```python
from build123d import *

# Parameters (mm, degrees)
F0_W     = 105
F0_H     = 85
F0_R     = 4
F1_DEPTH = 8
F2_D     = 9
F2_DEPTH = 14
F2_TIP   = 2.7038727856


with BuildPart() as f1:
    # F0 (on Top) → F1 (new body)
    with BuildSketch(Plane.XY):
        Rectangle(F0_W, F0_H)
        with Locations((-42.5, -30)):
            Circle(F0_R, mode=Mode.SUBTRACT)
        with Locations((42.5, -30)):
            Circle(F0_R, mode=Mode.SUBTRACT)
        with Locations((-42.5, 30)):
            Circle(F0_R, mode=Mode.SUBTRACT)
        with Locations((42.5, 30)):
            Circle(F0_R, mode=Mode.SUBTRACT)
        with Locations((-42.5, 30)):
            Circle(F0_R)
        with Locations((42.5, 30)):
            Circle(F0_R)
        with Locations((42.5, -30)):
            Circle(F0_R)
        with Locations((-42.5, -30)):
            Circle(F0_R)
    extrude(amount=F1_DEPTH)

    # F2
    with Locations(Plane(origin=(0, 0, 0), x_dir=(1, 0, 0), z_dir=(0, 0, -1))):
        with Locations((-42.5, -30), (42.5, -30), (42.5, 30), (-42.5, 30)):
            Hole(F2_D / 2, depth=F2_DEPTH)
            with Locations((0, 0, -(F2_DEPTH + F2_TIP / 2))):  # 118° drill point
                Cone(0, F2_D / 2, F2_TIP, mode=Mode.SUBTRACT)


solid = f1.part
```
Geometry check sheet. Reference: the model listing, model coordinates, mm. Coordinates: 2 decimals unless noted, no trailing zeros. Write each loop counter-clockwise with the first axis right and the second up, starting at its lowest first coordinate (ties: lowest second). Pieces come first, ordered by that corner, then holes. Notation, with made-up numbers: (22.5, 74) -> (49.5, 74) arc R19 cw to (49.5, 89) -> close; hole circle Ø11 at (85, 50.5). An arc over 180 degrees is marked (long way). Use CSV: the item, a comma, the result in double quotes. Start each with the question number.
Item 1: Cross-section at C-C, the plane z = 3.25. Record the cut outline in (x, y).
Item 2: Cross-section at B-B, the plane x = -42.5. Record the cut outline in (y, z), plus the area to 3 significant figures.
Item 3: Mould release check, pull along Y, two halves, no side actions. Record for faces 1 (the cylindrical face through (38.34, 31.72, 4.06)), 2 (the flat face through (-1, -42.5, 4)), 3 (the flat face through (-1, 1, 8)): released by +Y, released by -Y, zero draft, split by the parting line, or undercut.
Item 4: Cross-section at A-A, the plane y = 30. Record the cut outline in (x, z).
Item 5: Thickness scan on line 1 (X direction, y = -30, z = 2.75); line 2 (Y direction, x = -42.5, z = 4); line 3 (Y direction, x = 45.5, z = 3.5). Record the ranges inside material, lowest first.
Answers:
1,outline,"(-52.5, -42.5) -> (52.5, -42.5) -> (52.5, 42.5) -> (-52.5, 42.5) -> close; hole circle Ø9 at (-42.5, -30); hole circle Ø9 at (-42.5, 30); hole circle Ø9 at (42.5, -30); hole circle Ø9 at (42.5, 30)"
2,outline,"(-42.5, 0) -> (-34.5, 0) -> (-34.5, 8) -> (-42.5, 8) -> close; (-25.5, 0) -> (25.5, 0) -> (25.5, 8) -> (-25.5, 8) -> close; (34.5, 0) -> (42.5, 0) -> (42.5, 8) -> (34.5, 8) -> close"
2,area,"536 mm^2"
3,face 1,"undercut"
3,face 2,"released by -Y"
3,face 3,"zero draft"
4,outline,"(-52.5, 0) -> (-47, 0) -> (-47, 8) -> (-52.5, 8) -> close; (-38, 0) -> (38, 0) -> (38, 8) -> (-38, 8) -> close; (47, 0) -> (52.5, 0) -> (52.5, 8) -> (47, 8) -> close"
5,line 1,"-52.5 to -47, -38 to 38, 47 to 52.5"
5,line 2,"-42.5 to -34.5, -25.5 to 25.5, 34.5 to 42.5"
5,line 3,"-42.5 to -33.35, -26.65 to 26.65, 33.35 to 42.5"
